Geometry: final body of the model. Coordinates: model frame, mm. A direction names the side the tool comes from. Round coordinates to 2 decimals unless told otherwise and drop trailing zeros. Loops run counter-clockwise (first coordinate to the right, second up) from the corner with the lowest first, then second, coordinate; pieces in that order, holes last. Notation, with made-up numbers: (-26, 68.5) -> (22, 68.5) arc R9 ccw to (22, 81.5) -> close; hole circle Ø1 at (-23, -35). An arc over 180 degrees is marked (long way). Answer in a Markdown table with one row per item.
Autodesk Inventor part; units mm, degrees
ref_plane "YZ Plane" through (0, 0, 0) normal (1, 0, 0) x (0, 1, 0)
ref_plane "XZ Plane" through (0, 0, 0) normal (0, 1, 0) x (-1, 0, 0)
ref_plane "XY Plane" through (0, 0, 0) normal (0, 0, 1) x (1, 0, 0)
sketch "Esboço10" plane through (0, 0, 0) normal (1, 0, 0) x (0, 1, 0)
  line L0 (0, 0) -> (0, 17.5)
  line L1 (0, 0) -> (0, -17.5)
  line L2 (0, 17.5) -> (3, 17.5)
  circle A0 centre (8, 0) radius 2.5
  circle A1 centre (8, 0) radius 7.5
  line L3 (3, 17.5) -> (3, 5.5902)
  line L4 (0, -17.5) -> (3, -17.5)
  line L5 (3, -17.5) -> (3, -5.5902)
  dimension "d67" = 17.5
  dimension "d68" = 17.5
  dimension "d69" = 3
  dimension "d70" = 5
  dimension "d71" = 15
  dimension "d93" = 3
  dimension "d94" = 0
  dimension "d97" = 8
extrude "Extrusão7" add sketch "Esboço10" along normal mid plane 30
fillet "Arredondamento5" radius 2 2 edges at (0, 3, 5.5902) (0, 3, -5.5902)
fillet "Arredondamento6" radius 4 4 edges at (15, 1.5, 17.5) (15, 1.5, -17.5) (-15, 1.5, 17.5) (-15, 1.5, -17.5)
sketch "Esboço15" plane through (15, 0, 0) normal (1, 0, 0) x (0, 0, -1)
  line L0 (13.5, 3) -> (13.5, 0)
  line L1 (13.5, 3) -> (9.0139, 3)
  arc A0 (7.1162, 5.6316) -> (9.0139, 3) centre (9.0139, 5) ccw
  arc A1 (7.1162, 5.6316) -> (-7.1162, 5.6316) centre (0, 8) ccw
  arc A2 (-9.0139, 3) -> (-7.1162, 5.6316) centre (-9.0139, 5) ccw
  line L2 (-9.0139, 3) -> (-13.5, 3)
  line L3 (-13.5, 0) -> (-13.5, 3)
  line L4 (-13.5, 0) -> (13.5, 0)
  circle A3 centre (0, 8) radius 2.5
  circle A4 centre (0, 8) radius 5.5
  point P0 (0, 0)
  dimension "d98" = 11
extrude "Extrusão11" cut sketch "Esboço15" against normal blind 4 contours A4
mirror "Espelhar1" about plane through (0, 0, 0) normal (1, 0, 0) of "Extrusão11"
equation "\"d68\" = d67"
properties part number "encaixeBase"
Item 1: Cut plane B-B (y = 8). Output: boundary loops of the cut face in (x, z), then the cut area to 3 significant figures.
Answer:
| item | result |
|---|---|
| outline | (-15, -7.5) -> (15, -7.5) -> (15, -5.5) -> (11, -5.5) -> (11, -2.5) -> (-11, -2.5) -> (-11, -5.5) -> (-15, -5.5) -> close; (-15, 5.5) -> (-11, 5.5) -> (-11, 2.5) -> (11, 2.5) -> (11, 5.5) -> (15, 5.5) -> (15, 7.5) -> (-15, 7.5) -> close |
| area | 252 mm² |
Item 2: Cut plane A-A (z = 0). Output: boundary loops of the cut face in (x, y).
Answer:
| item | result |
|---|---|
| outline | (-15, 0) -> (15, 0) -> (15, 2.5) -> (11, 2.5) -> (11, 5.5) -> (-11, 5.5) -> (-11, 2.5) -> (-15, 2.5) -> close; (-15, 13.5) -> (-11, 13.5) -> (-11, 10.5) -> (11, 10.5) -> (11, 13.5) -> (15, 13.5) -> (15, 15.5) -> (-15, 15.5) -> close |
Item 3: Cut plane C-C (x = 3). Output: boundary loops of the cut face in (y, z).
Answer:
| item | result |
|---|---|
| outline | (0, -17.5) -> (3, -17.5) -> (3, -9.01) arc R2 cw to (5.63, -7.12) arc R7.5 ccw (long way) to (5.63, 7.12) arc R2 cw to (3, 9.01) -> (3, 17.5) -> (0, 17.5) -> close; hole circle Ø5 at (8, 0) |
Item 4: Reachability of faces 4 (the face through (-11, 8, -3)), 5 (the face through (13.03, 2.63, 1.19)), 6 (the face through (0, 3, 13)), 7 (the face through (0, 3, -13)) from +Z, -Z, +X, -X, +Y, -Y: full face, straight path, thin tool, end or side. Return the list, or none.
Answer:
| item | result |
|---|---|
| face 4 | -X |
| face 5 | +X |
| face 6 | +Z, +X, -X, +Y |
| face 7 | -Z, +X, -X, +Y |
Item 5: Pin query (flat end, axial travel): pin 1 Ø5 at (y, z) = (13.5, 5.5) entering from +X; pin 2 Ø2.5 at (x, z) = (-1.5, 15) entering from +Y; pin 3 Ø5 at (x, z) = (-1, 8) entering from +Y; pin 4 Ø3 at (x, z) = (0, -3) entering from +Y. Return the tip coordinate at first contact, or that it passes through.
Answer:
| item | result |
|---|---|
| pin 1 | stops at x = 15 |
| pin 2 | stops at y = 3 |
| pin 3 | stops at y = 13.1 |
| pin 4 | stops at y = 15.35 |
Item 6: Draft query along Z for faces 1 (the face through (13.859, 1.521, -16.297)), 2 (the face through (-15, 2, 0)), 3 (the face through (11, 8, 3)). Return one class per face: pulls with the +Z half, pulls with the -Z half, needs draft (parallel to the pull), parting line crosses it, or undercut.
Answer:
| item | result |
|---|---|
| face 1 | pulls with the -Z half |
| face 2 | needs draft |
| face 3 | undercut |
Item 7: Line query: probe 1 along Y at (x, z) = (-13.45, 0); probe 2 along Y at (x, z) = (6, 0); probe 3 along Z at (x, y) = (6.5, 8). Output: solid intervals per line, ascending. Write a range as [from, to].
Answer:
| item | result |
|---|---|
| probe 1 | y = [0, 2.5], [13.5, 15.5] |
| probe 2 | y = [0, 5.5], [10.5, 15.5] |
| probe 3 | z = [-7.5, -2.5], [2.5, 7.5] |
Item 8: Cut plane D-D (z = -11). Output: boundary loops of the cut face in (x, y).
Answer:
| item | result |
|---|---|
| outline | (-15, 0) -> (15, 0) -> (15, 3) -> (-15, 3) -> close |
